CAD build for the part. Positions are in the model's coordinates, mm. A direction names the side the tool comes from. Coordinates: 2 decimals unless noted, no trailing zeros. Write each loop counter-clockwise with the first axis right and the second up, starting at its lowest first coordinate (ties: lowest second). Pieces come first, ordered by that corner, then holes. Notation, with made-up numbers: (88, 38.25) - (146, 38.25) arc R22 cw to (146, 71.25) - close; hole circle Ø2 at (-13, 84.5). An arc over 180 degrees is marked (long way). One line per question, with ' | ' between items. Start each with the question number.
1. Band-saw the part on D-D, the plane y = 9. Write the cut outline in (x, z).
2. Two-plate mould, pull along Y, no slides. Class faces 6 (the flat face through (29, 27.25, -1)), 7 (the flat face through (2.75, 8, -1)), 8 (the flat face through (2, -1, -3)): +Y half, -Y half, draft (parallel to the pull), parting line (faces both ways), or undercut.
3. Flat gauge pins, fed straight in: P1, Ø4, axis at x = 25, y = 20, coming from the +Z side; P2, Ø1.8, axis at x = 47, z = -2.5, coming from the -Y side; P3, Ø3, axis at x = 1.5, z = -4, coming from the -Y side. Where does each tip first touch, or does it go through?
4. Band-saw the part on A-A, the plane x = 25. Write the cut outline in (y, z).
5. Which spindle directions (+Z, -Z, +X, -X, +Y, -Y) get a long thin tool onto all of the face, cutting with end or side? Do faces 1 (the flat face through (1, -20, -3)), 2 (the flat face through (48, -23, -3)), 3 (the flat face through (30, -27.25, -1)), 4 (the flat face through (56, -24, -3)), 5 (the flat face through (2.75, -9, -1)). Say none if no direction does.
6. Probe line 1 (Y direction, x = 25, z = -0.25); line 2 (Y direction, x = 25, z = 1.25); line 3 (X direction, y = 20, z = -0.5). List the from-to ranges inside material, lowest first.
7. Band-saw the part on B-B, the plane z = -2.5. Write the cut outline in (x, y).
8. Band-saw the part on C-C, the plane x = 33. Write the cut outline in (y, z).
from build123d import *

# Parameters (mm, degrees)
PAD007_DEPTH    = 30
PAD004_DEPTH    = 1.5
PAD006_DEPTH    = 2
SKETCH016_R     = 1.75
POCKET009_DEPTH = 2.5
SKETCH018_W     = 10
SKETCH018_H     = 2
SKETCH018_W_2   = 16
PAD008_DEPTH    = 4
CHAMFER001_SIZE = 1.5
CHAMFER002_SIZE = 1
CHAMFER003_SIZE = 0.5


with BuildPart() as part:
    # Sketch017 → Pad007 (new body, symmetric)
    with BuildSketch(Plane.XZ):
        Polygon((0, 0), (0, 2), (58, 2), (60, 0), align=None)
    extrude(amount=PAD007_DEPTH, both=True)

    # Sketch013 → Pad004 (join)
    with BuildSketch(Plane.XY):
        with BuildLine():
            ThreePointArc((3.75, 27.25), (3.042893, 26.957107), (2.75, 26.25))
            Line((2.75, 21), (2.75, 26.25))
            Line((0, 21), (2.75, 21))
            Line((0, 15), (0, 21))
            Line((2.75, 15), (0, 15))
            Line((2.75, 2), (2.75, 15))
            Line((0, 2), (2.75, 2))
            Line((0, -4), (0, 2))
            Line((2.75, -4), (0, -4))
            Line((2.75, -14), (2.75, -4))
            Line((0, -14), (2.75, -14))
            Line((0, -20), (0, -14))
            Line((2.75, -20), (0, -20))
            Line((2.75, -26.25), (2.75, -20))
            ThreePointArc((2.75, -26.25), (3.042893, -26.957107), (3.75, -27.25))
            Line((55.25, -27.25), (3.75, -27.25))
            ThreePointArc((55.25, -27.25), (55.957107, -26.957107), (56.25, -26.25))
            Line((56.25, 26.25), (56.25, -26.25))
            ThreePointArc((56.25, 26.25), (55.957107, 26.957107), (55.25, 27.25))
            Line((3.75, 27.25), (55.25, 27.25))
        make_face()
    extrude(amount=-PAD004_DEPTH)

    # Sketch015 → Pad006 (join)
    with BuildSketch(Plane.YZ):
        with BuildLine():
            ThreePointArc((-14, -5.354249), (-17, -4), (-20, -5.354249))
            Line((-20, -5.354249), (-20, 0))
            Line((-20, 0), (-14, 0))
            Line((-14, 0), (-14, -5.354249))
        make_face()
        with BuildLine():
            ThreePointArc((2, -5.645898), (-1, -4.5), (-4, -5.645898))
            Line((-4, -5.645898), (-4, 0))
            Line((-4, 0), (2, 0))
            Line((2, 0), (2, -5.645898))
        make_face()
        with BuildLine():
            ThreePointArc((21, -5.645898), (18, -4.5), (15, -5.645898))
            Line((15, -5.645898), (15, 0))
            Line((15, 0), (21, 0))
            Line((21, 0), (21, -5.645898))
        make_face()
    extrude(amount=PAD006_DEPTH)

    # Sketch016 → Pocket009 (cut, symmetric)
    with BuildSketch(Plane.XY):
        with Locations((25, 20)):
            Circle(SKETCH016_R)
        with Locations((25, -20)):
            Circle(SKETCH016_R)
    extrude(amount=POCKET009_DEPTH, both=True, mode=Mode.SUBTRACT)

    # Sketch018 → Pad008 (join)
    with BuildSketch(Plane.XY.offset(-5)):
        with Locations((24, -24)):
            Rectangle(SKETCH018_W, SKETCH018_H)
        with Locations((48, -24)):
            Rectangle(SKETCH018_W_2, SKETCH018_H)
    extrude(amount=PAD008_DEPTH)

    # Chamfer001
    chamfer001_edges = [part.edges().sort_by_distance(p)[0] for p in [
        (23.25, 20, 2),
        (23.25, -20, 2),
    ]]
    chamfer(chamfer001_edges, length=CHAMFER001_SIZE)

    # Chamfer002
    chamfer002_edges = [part.edges().sort_by_distance(p)[0] for p in [
        (59, -30, 1),
        (0, -30, 1),
        (0, 30, 1),
        (59, 30, 1),
    ]]
    chamfer(chamfer002_edges, length=CHAMFER002_SIZE)

    # Chamfer003
    chamfer003_edges = [part.edges().sort_by_distance(p)[0] for p in [
        (28.792893, 30, 2),
        (0.5, 29.5, 2),
        (0, 0, 2),
        (0.5, -29.5, 2),
        (28.792893, -30, 2),
        (57.292893, -29.5, 2),
        (58, 0, 2),
        (57.292893, 29.5, 2),
    ]]
    chamfer(chamfer003_edges, length=CHAMFER003_SIZE)


solid = part.part
Filled in:
1) outline: (0, 0) - (2.75, 0) - (2.75, -1.5) - (56.25, -1.5) - (56.25, 0) - (60, 0) - (58.35, 1.65) - (57.5, 2) - (0.5, 2) - (0, 1.5) - close
2) face 6: +Y half | face 7: undercut | face 8: draft
3) P1: stops at z = 0.75 | P2: stops at y = -25 | P3: stops at y = -20
4) outline: (-30, 0) - (-27.25, 0) - (-27.25, -1.5) - (-25, -1.5) - (-25, -5) - (-23, -5) - (-23, -1.5) - (-21.75, -1.5) - (-21.75, 0.5) - (-23.25, 2) - (-29.5, 2) - (-30, 1.5) - close; (-18.25, -1.5) - (18.25, -1.5) - (18.25, 0.5) - (16.75, 2) - (-16.75, 2) - (-18.25, 0.5) - close; (21.75, -1.5) - (27.25, -1.5) - (27.25, 0) - (30, 0) - (30, 1.5) - (29.5, 2) - (23.25, 2) - (21.75, 0.5) - close
5) face 1: -Z, -X, -Y | face 2: -Z, +X, -X, +Y | face 3: -Z, +X, -X, -Y | face 4: -Z, +X, +Y, -Y | face 5: -Z, -X
6) line 1: y = -27.25 to -21.75, -18.25 to 18.25, 21.75 to 27.25 | line 2: y = -30 to -22.5, -17.5 to 17.5, 22.5 to 30 | line 3: x = 0 to 23.25, 26.75 to 56.25
7) outline: (0, -20) - (2, -20) - (2, -14) - (0, -14) - close; (0, -4) - (2, -4) - (2, 2) - (0, 2) - close; (0, 15) - (2, 15) - (2, 21) - (0, 21) - close; (19, -25) - (29, -25) - (29, -23) - (19, -23) - close; (40, -25) - (56, -25) - (56, -23) - (40, -23) - close
8) outline: (-30, 0) - (-27.25, 0) - (-27.25, -1.5) - (27.25, -1.5) - (27.25, 0) - (30, 0) - (30, 1.5) - (29.5, 2) - (-29.5, 2) - (-30, 1.5) - close
